Verification items for the finished model (mm, model axes). Face numbers are marked on the shaded views. Round coordinates to 2 decimals unless told otherwise and drop trailing zeros. Loops run counter-clockwise (first coordinate to the right, second up) from the corner with the lowest first, then second, coordinate; pieces in that order, holes last. Notation, with made-up numbers: (-11.75, -21) -> (27.25, -21) arc R15 ccw to (27.25, -4) -> close; hole circle Ø2 at (-28.5, 19). An arc over 180 degrees is marked (long way). Write item = value, one per line. Start each with the question number.
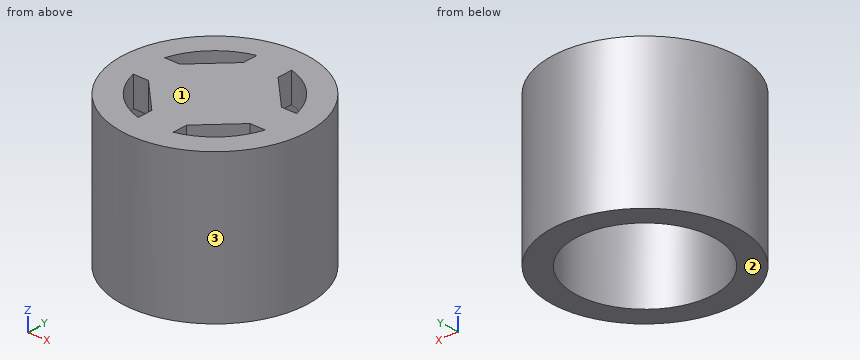
```python
from build123d import *

# Parameters (mm, degrees)
F0_R     = 3.15
F0_R_2   = 2.35
F1_DEPTH = 4
F2_R     = 3.15
F3_DEPTH = 1


# Not quite as in the source:
# - after a boolean that leaves OpenCascade's solid faulty, fix() repairs it


with BuildPart() as f1:
    # F0 (on Top) → F1 (new body)
    with BuildSketch(Plane.XY):
        Circle(F0_R)
        Circle(F0_R_2, mode=Mode.SUBTRACT)
    extrude(amount=F1_DEPTH)

    # F2 (on face) → F3 (join)
    with BuildSketch(Plane.XY.offset(4)):
        Circle(F2_R)
        with BuildLine():
            ThreePointArc((-2.2721135535, 0.6), (-1.6617009358, 1.6617009358), (-0.6, 2.2721135535))
            ThreePointArc((-0.6, 2.2721135535), (0, 2.35), (0.6, 2.2721135535))
            ThreePointArc((0.6, 2.2721135535), (1.6617009358, 1.6617009358), (2.2721135535, 0.6))
            ThreePointArc((2.2721135535, 0.6), (2.3304470441, 0.302517065), (2.35, 0))
            ThreePointArc((2.35, 0), (2.3304470441, -0.302517065), (2.2721135535, -0.6))
            ThreePointArc((2.2721135535, -0.6), (1.6617009358, -1.6617009358), (0.6, -2.2721135535))
            ThreePointArc((0.6, -2.2721135535), (0, -2.35), (-0.6, -2.2721135535))
            ThreePointArc((-0.6, -2.2721135535), (-1.6617009358, -1.6617009358), (-2.2721135535, -0.6))
            ThreePointArc((-2.2721135535, -0.6), (-2.35, 0), (-2.2721135535, 0.6))
        make_face(mode=Mode.SUBTRACT)
        with BuildLine():
            ThreePointArc((0.6, 2.2721135535), (0, 2.35), (-0.6, 2.2721135535))
            Line((-0.6, 2.2721135535), (-0.6, 1.75))
            Line((-0.6, 1.75), (-1.75, 0.6))
            Line((-1.75, 0.6), (-2.2721135535, 0.6))
            ThreePointArc((-2.2721135535, 0.6), (-2.35, 0), (-2.2721135535, -0.6))
            Line((-2.2721135535, -0.6), (-1.75, -0.6))
            Line((-1.75, -0.6), (-0.6, -1.75))
            Line((-0.6, -1.75), (-0.6, -2.2721135535))
            ThreePointArc((-0.6, -2.2721135535), (0, -2.35), (0.6, -2.2721135535))
            Line((0.6, -2.2721135535), (0.6, -1.75))
            Line((0.6, -1.75), (1.75, -0.6))
            Line((1.75, -0.6), (2.2721135535, -0.6))
            ThreePointArc((2.2721135535, -0.6), (2.3304470441, -0.302517065), (2.35, 0))
            ThreePointArc((2.35, 0), (2.3304470441, 0.302517065), (2.2721135535, 0.6))
            Line((2.2721135535, 0.6), (1.75, 0.6))
            Line((1.75, 0.6), (0.6, 1.75))
            Line((0.6, 1.75), (0.6, 2.2721135535))
        make_face()
    extrude(amount=F3_DEPTH)

    add(f1.part.fix(), mode=Mode.REPLACE)


solid = f1.part
```
(1) Section check C-C on y = -1. Enter the section's corners in (x, z).
(2) Section check D-D on y = 0. Enter the section's corners in (x, z), then the cut area to 3 significant figures.
(3) Scan lines: line 1 (Y direction, x = 0, z = 1.25); line 2 (X direction, y = -1, z = 4.5); line 3 (X direction, y = 1.25, z = 1.95). Record each from-to range of solid material in increasing order. Write a range as [from, to].
(4) Draft check along Z on the marked faces 1, 2 and 3. Enter one of: +Z half, -Z half, draft (parallel to the pull), parting line (faces both ways), or undercut.
(5) Section check A-A on z = 4.2. Enter the section's corners in (x, y).
(6) Depth check by flat-ended pin: pin 1 Ø0.6 at (x, z) = (-2, 4.5) entering from -Y; pin 2 Ø1.5 at (x, z) = (-1.5, 2) entering from +Y. Enter the tip coordinate at first touch or a pass-through.
(7) Section check B-B on x = -2. Enter the section's corners in (y, z), then the cut area to 3 significant figures.
Computed values:
q1.outline = (-2.99, 0) -> (-2.13, 0) -> (-2.13, 5) -> (-2.99, 5) -> close; (-1.35, 4) -> (1.35, 4) -> (1.35, 5) -> (-1.35, 5) -> close; (2.13, 0) -> (2.99, 0) -> (2.99, 5) -> (2.13, 5) -> close
q2.outline = (-3.15, 0) -> (-2.35, 0) -> (-2.35, 4) -> (2.35, 4) -> (2.35, 0) -> (3.15, 0) -> (3.15, 5) -> (-3.15, 5) -> close
q2.area = 12.7 mm²
q3.line_1 = [-3.15, -2.35], [2.35, 3.15]
q3.line_2 = [-2.99, -2.13], [-1.35, 1.35], [2.13, 2.99]
q3.line_3 = [-2.89, -1.99], [1.99, 2.89]
q4.face_1 = +Z half
q4.face_2 = -Z half
q4.face_3 = draft
q5.outline = circle Ø6.3 at (0, 0); hole (-2.27, -0.6) arc R2.35 ccw to (-0.6, -2.27) -> (-0.6, -1.75) -> (-1.75, -0.6) -> close; hole (-2.27, 0.6) -> (-1.75, 0.6) -> (-0.6, 1.75) -> (-0.6, 2.27) arc R2.35 ccw to start; hole (0.6, -2.27) arc R2.35 ccw to (2.27, -0.6) -> (1.75, -0.6) -> (0.6, -1.75) -> close; hole (0.6, 1.75) -> (1.75, 0.6) -> (2.27, 0.6) arc R2.35 ccw to (0.6, 2.27) -> close
q6.pin_1 = -2.65
q6.pin_2 = 3.06
q7.outline = (-2.43, 0) -> (-1.23, 0) -> (-1.23, 5) -> (-2.43, 5) -> close; (-0.6, 4) -> (0.6, 4) -> (0.6, 5) -> (-0.6, 5) -> close; (1.23, 0) -> (2.43, 0) -> (2.43, 5) -> (1.23, 5) -> close
q7.area = 13.2 mm²
